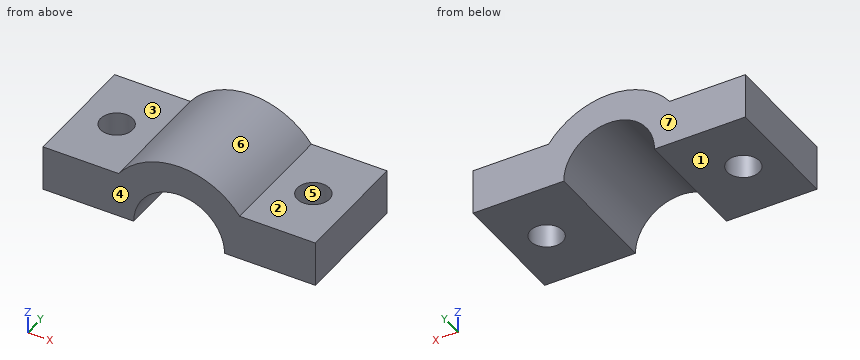
Autodesk Inventor part; units mm, degrees
ref_plane "YZ Plane" through (0, 0, 0) normal (1, 0, 0) x (0, 1, 0)
ref_plane "XZ Plane" through (0, 0, 0) normal (0, 1, 0) x (-1, 0, 0)
ref_plane "XY Plane" through (0, 0, 0) normal (0, 0, 1) x (1, 0, 0)
sketch "Sketch1" plane through (0, 0, 0) normal (0, 1, 0) x (-1, 0, 0)
  line L0 (0, 0) -> (0, 38.1) construction
  line L1 (0, 0) -> (0, -38.1) construction
  arc A0 (-9.525, -38.1) -> (9.525, -38.1) centre (0, -38.1) ccw construction
  circle A1 centre (0, 38.1) radius 9.525 construction
  line L2 (15.875, -38.1) -> (28.575, -38.1)
  line L3 (15.875, -38.1) -> (-15.875, -38.1) construction
  line L4 (15.875, -38.1) -> (9.525, -38.1)
  line L5 (-9.525, -38.1) -> (-15.875, -38.1)
  arc A2 (9.525, -38.1) -> (-9.525, -38.1) centre (0, -38.1) ccw construction
  arc A3 (12.7, -28.575) -> (-12.7, -28.575) centre (0, -38.1) ccw
  arc A4 (9.525, -38.1) -> (-9.525, -38.1) centre (0, -38.1) ccw
  line L6 (28.575, -38.1) -> (28.575, -28.575)
  line L7 (28.575, -28.575) -> (12.7, -28.575)
  line L8 (-15.875, -38.1) -> (-28.575, -38.1)
  line L9 (-28.575, -38.1) -> (-28.575, -28.575)
  line L10 (-28.575, -28.575) -> (-12.7, -28.575)
  point P0 (-101.6, -47.625)
  dimension "d0" = 76.2
  dimension "d1" = 19.05
  dimension "d9" = 9.525
  dimension "d17" = 15.875
  dimension "d18" = 15.875
extrude "Extrusion1" add sketch "Sketch1" along normal mid plane 25.4
sketch "Sketch2" plane through (-28.575, 12.7, -28.575) normal (0, 0, 1) x (1, 0, 0)
  line L0 (19.05, 0) -> (0, 0) construction
  line L1 (15.875, -25.4) -> (15.875, 0) construction
  line L2 (0, 0) -> (15.875, -25.4) construction
  line L3 (15.875, -25.4) -> (0, -25.4) construction
  line L4 (15.875, 0) -> (0, -25.4) construction
  point P0 (28.575, -12.7)
  point P1 (7.9375, -12.7)
hole "Hole1" at (-20.6375, 0, -28.575) direction (0, 0, -1) diameter 6.7564 end through all
sketch "Sketch3" plane through (12.7, 12.7, -28.575) normal (0, 0, 1) x (1, 0, 0)
  line L0 (0, -25.4) -> (0, 0) construction
  line L1 (15.875, -25.4) -> (15.875, 0) construction
  line L2 (0, 0) -> (15.875, -25.4) construction
  line L3 (15.875, -25.4) -> (15.875, 0) construction
  line L4 (15.875, 0) -> (0, -25.4) construction
  point P0 (-12.7, -12.7)
  point P1 (7.9375, -12.7)
hole "Hole2" at (20.6375, 0, -28.575) direction (0, 0, -1) diameter 6.7564 end through all
equation "\"d0\" = crutchTubSpacing"
equation "\"d1\" = cruchTubeDiam"
equation "\"cruchTubeDiam\" = 19.05"
equation "\"wallThickness\" = 6.35"
equation "\"crutchTubSpacing\" = 76.2"
equation "\"supportHeight\" = 25.4"
properties part number "innerCrutchAttacement"
Verification items for the finished model (mm, model axes). Face numbers are marked on the shaded views. A direction names the side the tool comes from. Give positions to 0.01 mm unless a question says otherwise; leave off trailing zeros. Order: outer loops, then holes, each group sorted by start corner. A loop starts at its lowest first (then second) coordinate and runs counter-clockwise, first axis right, second up. Notation, with made-up numbers: M -18.75,71.5 L -14.75,71.5 A21 ccw -14.75,92.5 Z; hole C 14,-37 d7. An arc over 180 degrees is marked long. Answer in a Markdown table with one row per item. Add a question column.
Item 1: Scan lines: probe 1 along Y at (x, z) = (20.5, -31); probe 2 along X at (y, z) = (0, -32.25) (3 decimals); probe 3 along X at (y, z) = (2, -34.5) (3 decimals). Record each from-to range of solid material in increasing order. Write a range as from..to.
Item 2: Section check B-B, the plane y = 0. Enter the section's corners in (x, z) (3 decimals), and give its area (3 significant figures).
Item 3: Section check D-D, the plane x = 0. Enter the section's corners in (y, z) (3 decimals), and give its area (3 significant figures).
Item 4: Mould release check, pull along Y, two halves, no side actions. Record for the marked faces 4, 5, 6 and 7: released by +Y, released by -Y, zero draft, split by the parting line, or undercut.
Item 5: Gauge pin test, flat ends, axial feed: pin 1 (1 mm diameter, centred on x = 5.5, y = -0.5, fed in from +Z); pin 2 (1 mm diameter, centred on x = -2.5, y = 2.5, fed in from +Z); pin 3 (8 mm diameter, centred on x = 22, y = 3.5, fed in from +Z) (3 decimals). Record the tip position at first contact, or that the pin passes through.
Item 6: Section check C-C, the plane z = -30.75. Enter the section's corners in (x, y) (1 decimal), and give its area (3 significant figures).
Item 7: Section check A-A, the plane z = -36.5. Enter the section's corners in (x, y) (1 decimal).
Item 8: Tool access check on the marked faces 1, 2 and 3. Record the directions out of +Z, -Z, +X, -X, +Y, -Y that give a thin tool (end or side, any length) a straight path to the whole face; none if there is none.
Filled sheet:
| question | item | result |
|---|---|---|
| 1 | probe 1 | y = -12.7..-3.38, 3.38..12.7 |
| 1 | probe 2 | x = -28.575..-24.016, -17.259..-7.517, 7.517..17.259, 24.016..28.575 |
| 1 | probe 3 | x = -28.575..-23.36, -17.915..-8.818, 8.818..17.915, 23.36..28.575 |
| 2 | outline | M -28.575,-38.1 L -24.016,-38.1 L -24.016,-28.575 L -28.575,-28.575 Z; M -17.259,-38.1 L -9.525,-38.1 A9.525 cw 9.525,-38.1 L 17.259,-38.1 L 17.259,-28.575 L 12.7,-28.575 A15.875 ccw -12.7,-28.575 L -17.259,-28.575 Z; M 24.016,-38.1 L 28.575,-38.1 L 28.575,-28.575 L 24.016,-28.575 Z |
| 2 | area | 386 mm^2 |
| 3 | outline | M -12.7,-28.575 L 12.7,-28.575 L 12.7,-22.225 L -12.7,-22.225 Z |
| 3 | area | 161 mm^2 |
| 4 | face 4 | released by -Y |
| 4 | face 5 | undercut |
| 4 | face 6 | zero draft |
| 4 | face 7 | released by +Y |
| 5 | pin 1 | stops at z = -23.03 |
| 5 | pin 2 | stops at z = -22.35 |
| 5 | pin 3 | stops at z = -28.575 |
| 6 | outline | M -28.6,-12.7 L -6.1,-12.7 L -6.1,12.7 L -28.6,12.7 Z; M 6.1,-12.7 L 28.6,-12.7 L 28.6,12.7 L 6.1,12.7 Z; hole C -20.6,0 d6.8; hole C 20.6,0 d6.8 |
| 6 | area | 1,070 mm^2 |
| 7 | outline | M -28.6,-12.7 L -9.4,-12.7 L -9.4,12.7 L -28.6,12.7 Z; M 9.4,-12.7 L 28.6,-12.7 L 28.6,12.7 L 9.4,12.7 Z; hole C -20.6,0 d6.8; hole C 20.6,0 d6.8 |
| 8 | face 1 | -Z, +X, -X, +Y, -Y |
| 8 | face 2 | +Z, +X, +Y, -Y |
| 8 | face 3 | +Z, -X, +Y, -Y |
